Read the model definition and answer for the solid it produces. Units are mm, in the model's axes. Face numbers are marked on the shaded views. A direction names the side the tool comes from. Coordinates: 2 decimals unless noted, no trailing zeros. Write each loop counter-clockwise with the first axis right and the second up, starting at its lowest first coordinate (ties: lowest second). Pieces come first, ordered by that corner, then holes. Notation, with made-up numbers: (78, 48) -> (113, 48) arc R13 cw to (113, 57) -> close; hole circle Ø2 at (-28.75, 73.25). An arc over 180 degrees is marked (long way). Use CSV: the item, a comma, the result in double quotes. Start each with the question number.
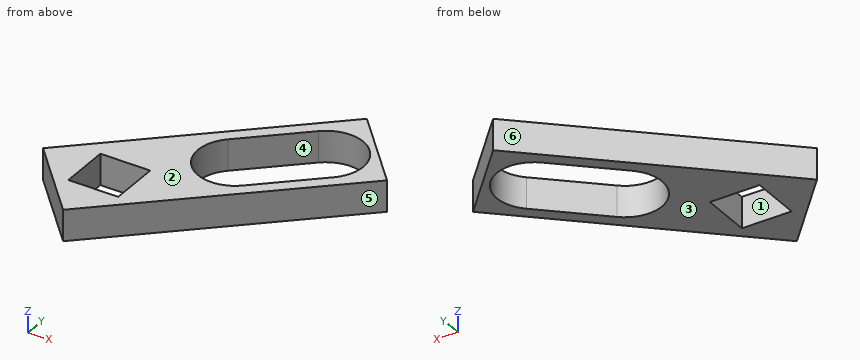
from build123d import *

# Parameters (mm, degrees)
BOSS_EXTRUDE1_DEPTH = 2.5
SKETCH2_W           = 4
SKETCH2_H           = 4
CUT_EXTRUDE1_DEPTH  = 27.670895226
CUT_EXTRUDE2_DEPTH  = 27.670895226


with BuildPart() as part:
    # Sketch1 → Boss-Extrude1 (new body)
    with BuildSketch(Plane.XY):
        Polygon((0, 0), (16.37938033, 15), (10.976408696, 20.899821821), (-5.402971634, 5.899821821), align=None)
    extrude(amount=BOSS_EXTRUDE1_DEPTH)

    # Sketch2 → Cut-Extrude1 (cut, through all)
    with BuildSketch(Plane.XY.offset(2.5)):
        with Locations((0.237599868, 5.405134804)):
            Rectangle(SKETCH2_W, SKETCH2_H)
    extrude(amount=-CUT_EXTRUDE1_DEPTH, mode=Mode.SUBTRACT)

    # Sketch3 → Cut-Extrude2 (cut, through all)
    with BuildSketch(Plane.XY.offset(2.5)):
        with BuildLine():
            Line((13.122836829, 13.373677638), (8.543100141, 9.179620906))
            ThreePointArc((8.543100141, 9.179620906), (4.304552595, 9.365939726), (4.490871415, 13.604487272))
            Line((4.490871415, 13.604487272), (9.070608103, 17.798544003))
            ThreePointArc((9.070608103, 17.798544003), (13.309155649, 17.612225183), (13.122836829, 13.373677638))
        make_face()
    extrude(amount=-CUT_EXTRUDE2_DEPTH, mode=Mode.SUBTRACT)


solid = part.part
1) Section C-C, the plane y = 11 is taken. Give the vertices of the cut face in (x, z), plus the area to 3 significant figures.
2) Which of the six approach directions +Z, -Z, +X, -X, +Y, -Y give full straight-line access (tool end or side, diameter ignored) to the marked faces 1 and 2?
3) Section A-A, the plane x = 1.75 is taken. Give the vertices of the cut face in (y, z), plus the area to 3 significant figures.
4) Find the intervals of material crossed by line 1 along X through (y, z) = (13.5, 1.8); line 2 along X through (y, z) = (12.25, 0.8); line 3 along Y through (x, z) = (7.75, 2.2), in increasing order.
5) Section B-B, the plane z = 0.4 is taken. Give the vertices of the cut face in (x, y).
6) The mould has two halves that part along X. Classify the marked faces 3, 4, 5 and 6: pulls with the +X half, pulls with the -X half, needs draft (parallel to the pull), parting line crosses it, or undercut.
7) Section D-D, the plane y = 2.25 is taken. Give the vertices of the cut face in (x, z), plus the area to 3 significant figures.
8) This flat-tipped pin is pushed along its axis until it touches: pin 1 (1.2 mm diameter, centred on y = 4.5, z = 1.5, fed in from +X). Where does it stop, or does it pass through?
The answers:
1,outline,"(0.17, 0) -> (3.54, 0) -> (3.54, 2.5) -> (0.17, 2.5) -> close; (10.53, 0) -> (12.01, 0) -> (12.01, 2.5) -> (10.53, 2.5) -> close"
1,area,"12.1 mm^2"
2,face 1,"+Z, -Z"
2,face 2,"+Z, +X, -X, +Y, -Y"
3,outline,"(1.6, 0) -> (3.41, 0) -> (3.41, 2.5) -> (1.6, 2.5) -> close; (7.41, 0) -> (12.45, 0) -> (12.45, 2.5) -> (7.41, 2.5) -> close"
3,area,"17.1 mm^2"
4,line 1,"x = 2.9 to 4.38, 13.25 to 14.74"
4,line 2,"x = 1.53 to 3.64, 11.9 to 13.38"
4,line 3,"y = 7.1 to 8.66, 16.59 to 17.95"
5,outline,"(-5.4, 5.9) -> (0, 0) -> (16.38, 15) -> (10.98, 20.9) -> close; hole (-1.76, 3.41) -> (2.24, 3.41) -> (2.24, 7.41) -> (-1.76, 7.41) -> close; hole (4.49, 13.6) arc R3 ccw to (8.54, 9.18) -> (13.12, 13.37) arc R3 ccw to (9.07, 17.8) -> close"
6,face 3,"needs draft"
6,face 4,"undercut"
6,face 5,"pulls with the +X half"
6,face 6,"pulls with the -X half"
7,outline,"(-2.06, 0) -> (2.46, 0) -> (2.46, 2.5) -> (-2.06, 2.5) -> close"
7,area,"11.3 mm^2"
8,pin 1,"stops at x = 5.57"
